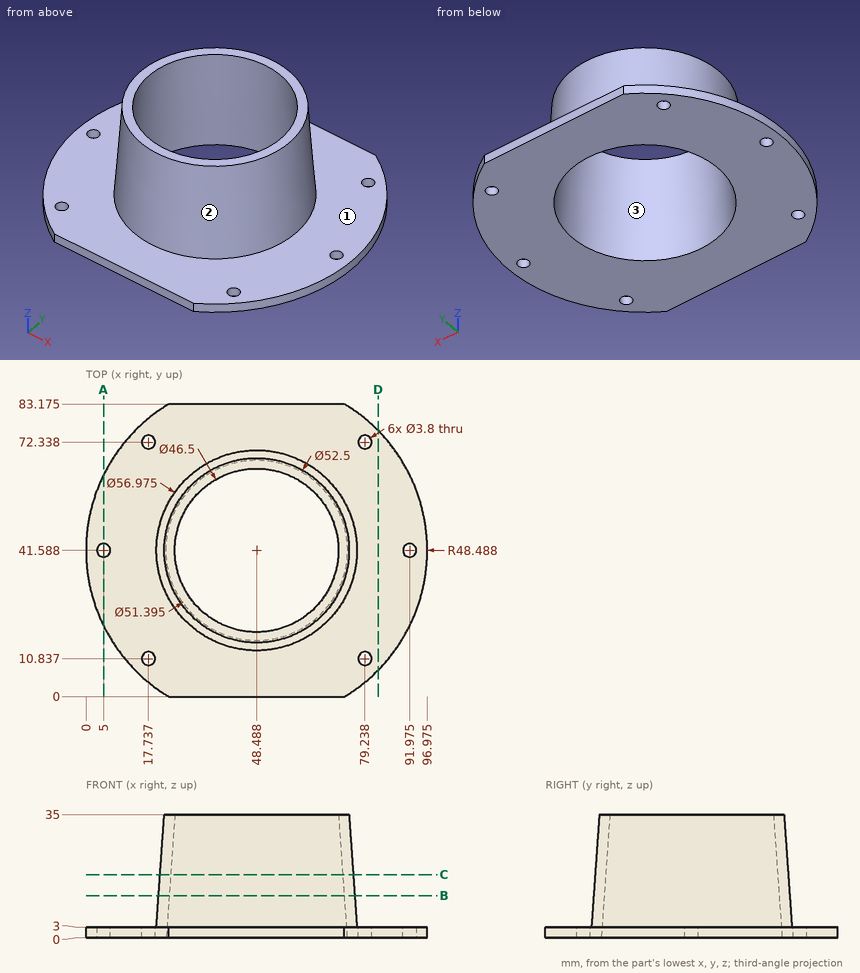
The figure shows three views and two pictorial views of one solid part (mm, origin at its lowest corner). Answer the questions. Coordinates: 2 decimals unless noted, no trailing zeros. Loops run counter-clockwise (first coordinate to the right, second up) from the corner with the lowest first, then second, coordinate; pieces in that order, holes last.
1) Find section D-D on x = 83. Write down the section's boundary in (y, z), then the cut area to 3 significant figures.
2) Find the intervals of material crossed by L1, parallel to Z at x = 79.5, y = 25; L2, parallel to X at y = 55.5, z = 7.5 (1 decimal); L3, parallel to X at y = 58, z = 6 (1 decimal), in increasing order.
3) Flat-ended cylindrical pins translate along their axes: pin 1 Ø6 at (y, z) = (11.5, 31.5) entering from +X; pin 2 Ø4 at (y, z) = (61, 4.5) entering from -X; pin 3 Ø4.5 at (x, y) = (79.24, 72.34) entering from +Z; pin 4 Ø6 at (y, z) = (53, 26) entering from -X (1 decimal). Find the tip coordinate at first contact, or state that the pin passes through.
4) Find section B-B on z = 12. Write down the section's boundary in (x, y), then the cut area to 3 significant figures.
5) Find section A-A on x = 5. Write down the section's boundary in (y, z), then the cut area to 3 significant figures.
6) Determine the mould class of the marked faces 1, 2 and 3 for opening direction X: pulls with the +X half, pulls with the -X half, needs draft (parallel to the pull), parting line crosses it, or undercut.
7) Find section C-C on z = 18. Write down the section's boundary in (x, y).
Values:
1. outline: (7.53, 0) - (75.65, 0) - (75.65, 3) - (7.53, 3) - close
1. area: 204 mm2
2. L1: z = 0 to 3
2. L2: x = 24 to 27.5, 69.5 to 73
2. L3: x = 25.5 to 29.3, 67.7 to 71.5
3. pin 1: passes through
3. pin 2: stops at x = 3.5
3. pin 3: stops at z = 3
3. pin 4: stops at x = 22.9
4. outline: circle Ø55.72 at (48.49, 41.59); hole circle Ø49.72 at (48.49, 41.59)
4. area: 497 mm2
5. outline: (20.14, 0) - (39.69, 0) - (39.69, 3) - (20.14, 3) - close; (43.49, 0) - (63.03, 0) - (63.03, 3) - (43.49, 3) - close
5. area: 117 mm2
6. face 1: needs draft
6. face 2: parting line crosses it
6. face 3: undercut
7. outline: circle Ø54.88 at (48.49, 41.59); hole circle Ø48.88 at (48.49, 41.59)
